from build123d import *

# Parameters (mm, degrees)
F1_DEPTH = 2
F2_W     = 7
F2_H     = 10
F2_H_2   = 4
F3_DEPTH = 2


with BuildPart() as f1:
    # F0 (on Top) → F1 (new body)
    with BuildSketch(Plane.XY):
        with BuildLine():
            Line((2.549947, -7.5), (22.5, -7.5))
            Line((22.5, -7.5), (22.5, 7.5))
            Line((22.5, 7.5), (-22.5, 7.5))
            Line((-22.5, 7.5), (-22.5, -7.5))
            Line((-22.5, -7.5), (-2.548188, -7.5))
            Line((-2.548188, -7.5), (-2.548188, -5.046103))
            ThreePointArc((-2.548188, -5.046103), (-0.039812, -2.400311), (2.549947, -4.966498))
            Line((2.549947, -4.966498), (2.549947, -7.5))
        make_face()
    extrude(amount=F1_DEPTH)

    # F2 (on face) → F3 (join)
    with BuildSketch(Plane.XY.offset(2)):
        with Locations((-19, -12.5)):
            Rectangle(F2_W, F2_H)
        with Locations((-19, -5.5)):
            Rectangle(F2_W, F2_H_2)
        with Locations((19, -12.5)):
            Rectangle(F2_W, F2_H)
        with Locations((19, -5.5)):
            Rectangle(F2_W, F2_H_2)
    extrude(amount=F3_DEPTH)


solid = f1.part
Work out the finished part from the listing and answer in its coordinate system (mm). A direction names the side the tool comes from. Give positions to 0.01 mm unless a question says otherwise; leave off trailing zeros. Order: outer loops, then holes, each group sorted by start corner. A loop starts at its lowest first (then second) coordinate and runs counter-clockwise, first axis right, second up. Notation, with made-up numbers: (18.25, 15) -> (64.25, 15) arc R35 ccw to (64.25, 54) -> close; hole circle Ø10 at (50, -18). An arc over 180 degrees is marked (long way). Answer as a JSON object with one key per item and string values. Group by question number.
1. Section D-D on x = 0 is taken. Determine the outline of the cut face in (y, z).
2. The mould has two halves that part along X. Classify faces 1 (the flat face through (-22.5, -5, 2)), 2 (the flat face through (-19, -17.5, 3)), 3 (the flat face through (-2.548, -6, 1)): released by +X, released by -X, zero draft, split by the parting line, or undercut.
3. Consider line 1 along X through (y, z) = (-8.5, 2.3); line 2 along X through (y, z) = (-7, 1.6); line 3 along Y through (x, z) = (6.5, 0.9). Determine where each line is inside the solid, lowest interval first. Write a range as [from, to].
4. Section A-A on y = -6.25 is taken. Determine the outline of the cut face in (x, z).
5. Section B-B on z = 3.25 is taken. Determine the outline of the cut face in (x, y).
6. Section C-C on y = -9.25 is taken. Determine the outline of the cut face in (x, z).
7. Flat-ended cylindrical pins translate along their axes: pin 1 Ø2 at (y, z) = (-10.5, 0.5) entering from -X; pin 2 Ø6 at (x, y) = (-5.5, -3.5) entering from +Z; pin 3 Ø1.6 at (x, z) = (9.5, 1) entering from -Y; pin 4 Ø0.6 at (x, z) = (-18, 3.5) entering from +Y. Find the tip coordinate at first contact, or state that the pin passes through.
8. A tool of negligible diameter and unlimited length cuts with its end or side. For faces 4 (the flat face through (-19, -3.5, 3)), 5 (the flat face through (15.5, -10, 3)), 6 (the flat face through (2.55, -6, 1)), 7 (the flat face through (12, -7.5, 1)), 8 (the flat face through (22.5, -5, 2)), from which of +Z, -Z, +X, -X, +Y, -Y can it reach the whole face along a straight path? Write none if from no direction.
Result sheet:
{
 "1": {"outline": "(-2.4, 0) -> (7.5, 0) -> (7.5, 2) -> (-2.4, 2) -> close"},
 "2": {"face 1": "released by -X", "face 2": "zero draft", "face 3": "undercut"},
 "3": {"line 1": "x = [-22.5, -15.5], [15.5, 22.5]", "line 2": "x = [-22.5, -2.55], [2.55, 22.5]", "line 3": "y = [-7.5, 7.5]"},
 "4": {"outline": "(-22.5, 0) -> (-2.55, 0) -> (-2.55, 2) -> (-15.5, 2) -> (-15.5, 4) -> (-22.5, 4) -> close; (2.55, 0) -> (22.5, 0) -> (22.5, 4) -> (15.5, 4) -> (15.5, 2) -> (2.55, 2) -> close"},
 "5": {"outline": "(-22.5, -17.5) -> (-15.5, -17.5) -> (-15.5, -3.5) -> (-22.5, -3.5) -> close; (15.5, -17.5) -> (22.5, -17.5) -> (22.5, -3.5) -> (15.5, -3.5) -> close"},
 "6": {"outline": "(-22.5, 2) -> (-15.5, 2) -> (-15.5, 4) -> (-22.5, 4) -> close; (15.5, 2) -> (22.5, 2) -> (22.5, 4) -> (15.5, 4) -> close"},
 "7": {"pin 1": "passes through", "pin 2": "stops at z = 2", "pin 3": "stops at y = -7.5", "pin 4": "stops at y = -3.5"},
 "8": {"face 4": "+Z, +X, -X, +Y", "face 5": "+Z, +Y, -Y", "face 6": "+Z, -Z, -Y", "face 7": "-Z, +X, -X, -Y", "face 8": "+Z, -Z, +X, +Y, -Y"}
}
